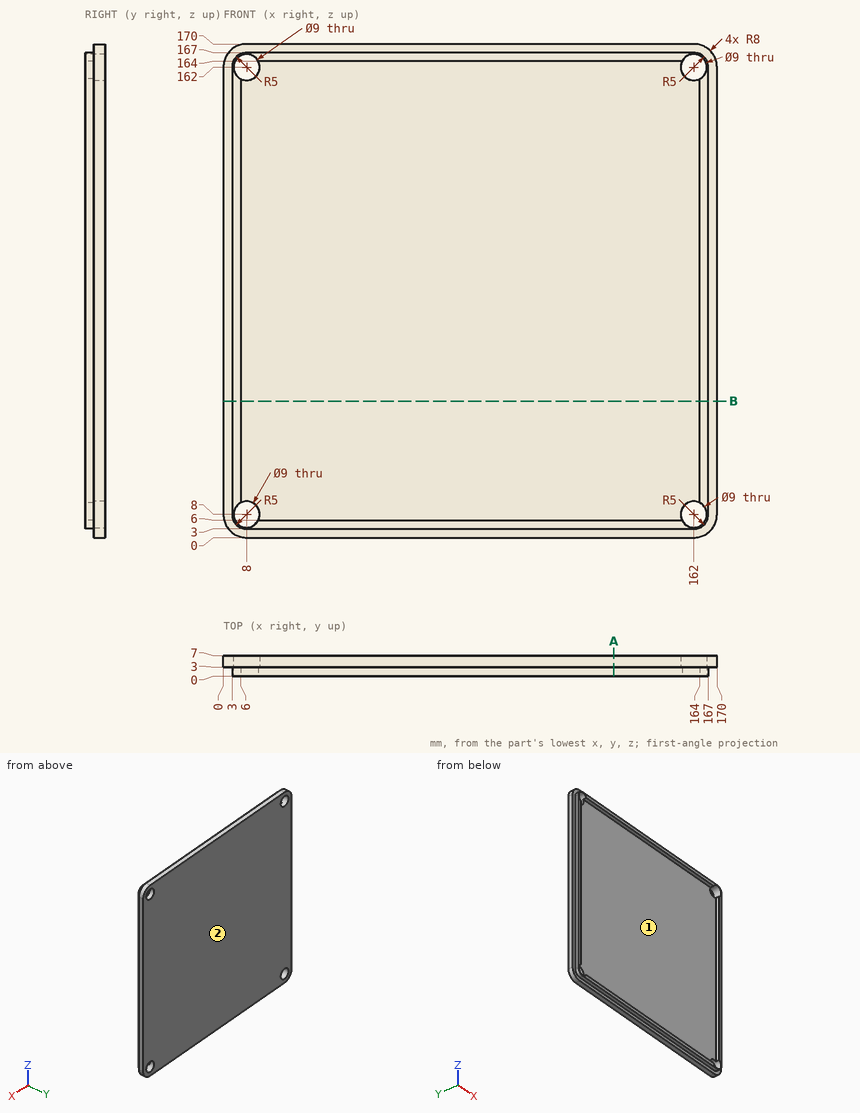
Geometry: see drawing. Coordinates: mm, zero at the bounding-box minimum. Coordinates: 2 decimals unless noted, no trailing zeros. Order: outer loops, then holes, each group sorted by start corner. A loop starts at its lowest first (then second) coordinate and runs counter-clockwise, first axis right, second up. Notation, with made-up numbers: M 73.25,44.5 L 103.25,44.5 A34 ccw 103.25,81.5 Z; hole C 38,88.5 d10. An arc over 180 degrees is marked long. Answer in a Markdown table with one row per item. Add a question column.
Q1. Section query B-B on z = 47. Return the cut outline in (x, y), and give its area (3 significant figures).
Q2. Mould query, pull axis X, two halves, no side actions, for the marked faces 1 and 2. Classes: released by +X, released by -X, zero draft, split by the parting line, or undercut.
Q3. Section query A-A on x = 134.5. Return the cut outline in (y, z).
Q4. Contact query for flat-ended pins moving along their axis: P1, Ø3.5, axis at x = 97.5, y = 1, coming from the +Z side; P2, Ø1.5, axis at y = 1.5, z = 82.5, coming from the -X side; P3, Ø2, axis at x = 92.5, z = 135, coming from the -Y side. Output: stop coordinate, or through.
Q5. Line query: L1, parallel to X at y = 4.25, z = 162; L2, parallel to Z at x = 8, y = 2.5. Output: solid intervals per line, ascending.
Completed:
| question | item | result |
|---|---|---|
| 1 | outline | M 0,3 L 3,3 L 3,0 L 6,0 L 6,3 L 164,3 L 164,0 L 167,0 L 167,3 L 170,3 L 170,7 L 0,7 Z |
| 1 | area | 698 mm2 |
| 2 | face 1 | undercut |
| 2 | face 2 | zero draft |
| 3 | outline | M 0,3 L 3,3 L 3,0 L 7,0 L 7,170 L 3,170 L 3,167 L 0,167 L 0,164 L 3,164 L 3,6 L 0,6 Z |
| 4 | P1 | stops at z = 167 |
| 4 | P2 | stops at x = 3 |
| 4 | P3 | stops at y = 3 |
| 5 | L1 | x = 0 to 3.5, 12.5 to 157.5, 166.5 to 170 |
| 5 | L2 | z = 3 to 3.5, 166.5 to 167 |
